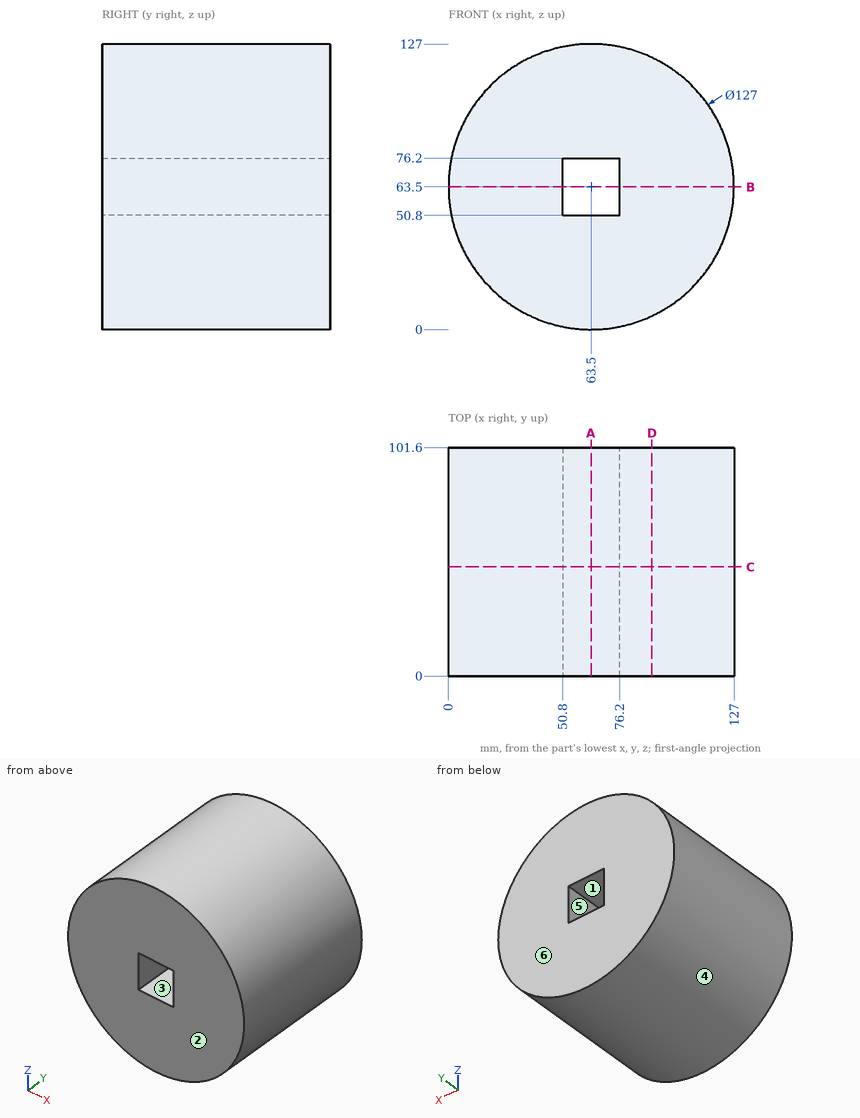
Geometry check sheet. Reference: drawing and pictorial views, mm from the part's lowest x, y, z. A direction names the side the tool comes from. Give positions to 0.01 mm unless a question says otherwise; leave off trailing zeros. Order: outer loops, then holes, each group sorted by start corner. A loop starts at its lowest first (then second) coordinate and runs counter-clockwise, first axis right, second up. Notation, with made-up numbers: M -35.75,70 L 22.25,70 A14 ccw 22.25,91 Z; hole C -36.5,37.5 d4. An arc over 180 degrees is marked long. Answer in a Markdown table with one row per item. Add a question column.
Item 1: Section check D-D, the plane x = 90.5. Enter the section's corners in (y, z), and give its area (3 significant figures).
Item 2: Section check A-A, the plane x = 63.5. Enter the section's corners in (y, z), and give its area (3 significant figures).
Item 3: Section check C-C, the plane y = 48.5. Enter the section's corners in (x, z), and give its area (3 significant figures).
Item 4: Section check B-B, the plane z = 63.5. Enter the section's corners in (x, y), and give its area (3 significant figures).
Item 5: Gauge pin test, flat ends, axial feed: pin 1 (20.5 mm diameter, centred on x = 59.5, y = 75, fed in from -Z); pin 2 (12.5 mm diameter, centred on x = 65.5, y = 62, fed in from +Z); pin 3 (4 mm diameter, centred on x = 80, y = 63.5, fed in from +Z). Record the tip position at first contact, or that the pin passes through.
Item 6: Scan lines: probe 1 along Z at (x, y) = (65.5, 68.5); probe 2 along Z at (x, y) = (68.5, 79); probe 3 along X at (y, z) = (13, 64). Record each from-to range of solid material in increasing order. Write a range as from..to.
Item 7: Tool access check on the marked faces 1 and 2. Record the directions out of +Z, -Z, +X, -X, +Y, -Y that give a thin tool (end or side, any length) a straight path to the whole face; none if there is none.
Item 8: Mould release check, pull along Z, two halves, no side actions. Record for the marked faces 3, 4, 5 and 6: released by +Z, released by -Z, zero draft, split by the parting line, or undercut.
Filled sheet:
| question | item | result |
|---|---|---|
| 1 | outline | M 0,6.03 L 101.6,6.03 L 101.6,120.97 L 0,120.97 Z |
| 1 | area | 11,700 mm^2 |
| 2 | outline | M 0,0 L 101.6,0 L 101.6,50.8 L 0,50.8 Z; M 0,76.2 L 101.6,76.2 L 101.6,127 L 0,127 Z |
| 2 | area | 10,300 mm^2 |
| 3 | outline | C 63.5,63.5 d127; hole M 50.8,50.8 L 76.2,50.8 L 76.2,76.2 L 50.8,76.2 Z |
| 3 | area | 12,000 mm^2 |
| 4 | outline | M 0,0 L 50.8,0 L 50.8,101.6 L 0,101.6 Z; M 76.2,0 L 127,0 L 127,101.6 L 76.2,101.6 Z |
| 4 | area | 10,300 mm^2 |
| 5 | pin 1 | stops at z = 0 |
| 5 | pin 2 | stops at z = 127 |
| 5 | pin 3 | stops at z = 125.32 |
| 6 | probe 1 | z = 0.03..50.8, 76.2..126.97 |
| 6 | probe 2 | z = 0.2..50.8, 76.2..126.8 |
| 6 | probe 3 | x = 0..50.8, 76.2..127 |
| 7 | face 1 | +Y, -Y |
| 7 | face 2 | +Z, -Z, +X, -X, -Y |
| 8 | face 3 | undercut |
| 8 | face 4 | split by the parting line |
| 8 | face 5 | undercut |
| 8 | face 6 | zero draft |
